Work out the finished part from the listing and answer in its coordinate system (mm). A direction names the side the tool comes from. Round coordinates to 2 decimals unless told otherwise and drop trailing zeros. Order: outer loops, then holes, each group sorted by start corner. A loop starts at its lowest first (then second) coordinate and runs counter-clockwise, first axis right, second up.
from build123d import *

# Parameters (mm, degrees)
F0_W     = 40
F0_H     = 200
F1_DEPTH = 330
F2_W     = 9
F2_H     = 25
F3_DEPTH = 25
F4_SIZE  = 5


with BuildPart() as f1:
    # F0 (on Top) → F1 (new body)
    with BuildSketch(Plane.XY):
        Rectangle(F0_W, F0_H)
    extrude(amount=F1_DEPTH)

    # F2 (on face) → F3 (cut)
    with BuildSketch(Plane(origin=(-20, 0, 0), x_dir=(0, -1, 0), z_dir=(-1, 0, 0))):
        Polygon((9, 25), (26, 25), (26, 275), (-26, 275), (-26, 25), (-9, 25), (0, 25), align=None)
        with Locations((4.5, 12.5)):
            Rectangle(F2_W, F2_H)
        with Locations((-4.5, 12.5)):
            Rectangle(F2_W, F2_H)
    extrude(amount=-F3_DEPTH, mode=Mode.SUBTRACT)

    # F4
    f4_edges = [f1.edges().sort_by_distance(p)[0] for p in [
        (-7.5, 9, 25),
        (-7.5, -9, 25),
    ]]
    chamfer(f4_edges, length=F4_SIZE)


solid = f1.part
Item 1: Find section B-B (x = 1). Write down the section's boundary in (y, z), plus the area to 3 significant figures.
Item 2: For a pull along Y with two mould halves and no side action, classify faces 4 (the face through (-8, 26, 152)), 5 (the face through (-8, 20, 25)), 6 (the face through (0, 100, 163)), 7 (the face through (9, 1, 0)) as released by +Y, released by -Y, zero draft, split by the parting line, or undercut.
Item 3: Find section A-A (y = 5.5). Write down the section's boundary in (x, z), plus the area to 4 significant figures.
Item 4: Find the intervals of material crossed by line 1 along Y through (x, z) = (4.5, 114); line 2 along Y through (x, z) = (-17.5, 15); line 3 along Z through (x, y) = (0, -20), in increasing order.
Item 5: Given pin 1 (12.5 mm diameter, centred on x = -6.5, y = -1.5, fed in from -Z), flat-ended and moving along its own axis, determine where the tip first touches the part or whether it passes through.
Item 6: Find section C-C (z = 114). Write down the section's boundary in (x, y), plus the area to 3 significant figures.
Item 7: A tool of negligible diameter and unlimited length cuts with its end or side. For faces 1 (the face through (20, -1, 163)), 2 (the face through (-8, 9, 10)), 3 (the face through (-8, 0, 275)), from which of +Z, -Z, +X, -X, +Y, -Y can it reach the whole face along a straight path? Write none if from no direction.
Model answer:
1. outline: (-100, 0) - (-9, 0) - (-9, 20) - (-14, 25) - (-26, 25) - (-26, 275) - (26, 275) - (26, 25) - (14, 25) - (9, 20) - (9, 0) - (100, 0) - (100, 330) - (-100, 330) - close
1. area: 52,500 mm2
2. face 4: undercut
2. face 5: undercut
2. face 6: released by +Y
2. face 7: zero draft
3. outline: (-20, 275) - (5, 275) - (5, 0) - (20, 0) - (20, 330) - (-20, 330) - close
3. area: 6,325 mm2
4. line 1: y = -100 to -26, 26 to 100
4. line 2: y = -100 to -9, 9 to 100
4. line 3: z = 0 to 25, 275 to 330
5. pin 1: stops at z = 275
6. outline: (-20, -100) - (20, -100) - (20, 100) - (-20, 100) - (-20, 26) - (5, 26) - (5, -26) - (-20, -26) - close
6. area: 6,700 mm2
7. face 1: +Z, -Z, +X, +Y, -Y
7. face 2: -Z, -X
7. face 3: -X
